Work out the finished part from the listing and answer in its coordinate system (mm). Face numbers are marked on the shaded views. A direction names the side the tool comes from. Give positions to 0.01 mm unless a question says otherwise; leave off trailing zeros. Loops run counter-clockwise (first coordinate to the right, second up) from the corner with the lowest first, then second, coordinate; pieces in that order, holes last. Notation, with made-up numbers: (-5, 12.25) - (1, 12.25) arc R19 ccw to (1, 24.25) - close; hole circle Ø5 at (14, -4.75). An arc over 180 degrees is marked (long way). One line per question, with ' | ' between items. Start each with the question number.
1. For a pull along X with two mould halves and no side action, classify the marked faces 4, 5 and 6 as released by +X, released by -X, zero draft, split by the parting line, or undercut.
2. Section B-B (y = 2.3) is taken. Determine the outline of the cut face in (x, z).
3. Find the intervals of material crossed by line 1 (Z direction, x = -28, y = 1.05); line 2 (Z direction, x = -18, y = 1.95); line 3 (X direction, y = 1.15, z = -0.5), in increasing order.
4. Which of the six approach directions +Z, -Z, +X, -X, +Y, -Y give full straight-line access (tool end or side, diameter ignored) to the marked faces 1, 2 and 3?
5. Each of these flat-tipped pins is pushed along its axis until it touches: pin 1 (0.8 mm diameter, centred on y = 2, z = 3.5, fed in from +X); pin 2 (0.8 mm diameter, centred on y = 1, z = 4.5, fed in from -X); pin 3 (1.8 mm diameter, centred on x = -8, z = 0, fed in from -Y); pin 4 (1.5 mm diameter, centred on x = -2, y = 1, fed in from +Z). Where does it stop, or does it pass through?
6. Section A-A (x = -18) is taken. Determine the outline of the cut face in (y, z), plus the area to 3 significant figures.
7. Section C-C (x = -8) is taken. Determine the outline of the cut face in (y, z).
Autodesk Inventor part; units mm, degrees
ref_plane "YZ Plane" through (0, 0, 0) normal (1, 0, 0) x (0, 1, 0)
ref_plane "XZ Plane" through (0, 0, 0) normal (0, 1, 0) x (-1, 0, 0)
ref_plane "XY Plane" through (0, 0, 0) normal (0, 0, 1) x (1, 0, 0)
sketch "Sketch1" plane through (0, 0, 0) normal (0, 1, 0) x (-1, 0, 0)
  line L0 (0, 0) -> (0, -3)
  line L1 (0, -3) -> (3, -3)
  line L2 (3, -3) -> (3, -5.5)
  line L3 (3, -5.5) -> (33, -5.5)
  line L4 (33, -5.5) -> (33, -3)
  line L5 (33, -3) -> (36, -3)
  line L6 (36, -3) -> (36, 3)
  line L7 (36, 3) -> (33, 3)
  line L8 (33, 3) -> (33, 5.5)
  line L9 (33, 5.5) -> (3, 5.5)
  line L10 (3, 5.5) -> (3, 3)
  line L11 (3, 3) -> (0, 3)
  line L12 (0, 3) -> (0, 0)
  circle A0 centre (28, 0) radius 1.5
  line L13 (0, 0) -> (8, 0)
  circle A1 centre (8, 0) radius 1.5
  arc A2 (17, -1.25) -> (19, -1.25) centre (18, -1.25) ccw
  arc A3 (19, 1.25) -> (17, 1.25) centre (18, 1.25) ccw
  line L14 (19, -1.25) -> (19, 1.25)
  line L15 (17, 1.25) -> (17, -1.25)
  arc A4 (22, -1.25) -> (24, -1.25) centre (23, -1.25) ccw
  arc A5 (24, 1.25) -> (22, 1.25) centre (23, 1.25) ccw
  line L16 (24, -1.25) -> (24, 1.25)
  line L17 (22, 1.25) -> (22, -1.25)
  dimension "d15" = 3
  dimension "d16" = 3
  dimension "d17" = 2.5
  dimension "d18" = 30
  dimension "d19" = 3
  dimension "d20" = 6
  dimension "d21" = 2.5
  dimension "d22" = 30
  dimension "d26" = 8
  dimension "d27" = 3
  dimension "d31" = 8
  dimension "d34" = 1
  dimension "d35" = 11
  dimension "d36" = 20
  dimension "d38" = 1
extrude "Extrusion1" add sketch "Sketch1" along normal blind 3
properties part number "Laser Mount Plate" material "Polycarbonate, Smoke"
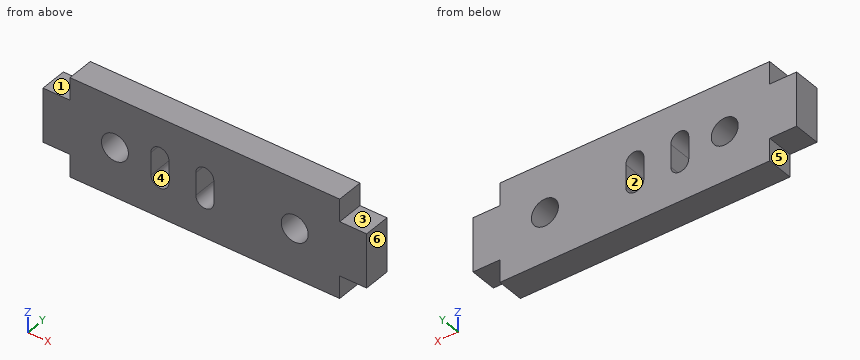
Conclusion:
1) face 4: undercut | face 5: released by -X | face 6: released by +X
2) outline: (-36, -3) - (-33, -3) - (-33, -5.5) - (-3, -5.5) - (-3, -3) - (0, -3) - (0, 3) - (-3, 3) - (-3, 5.5) - (-33, 5.5) - (-33, 3) - (-36, 3) - close; hole circle Ø3 at (-28, 0); hole (-24, -1.25) arc R1 ccw to (-22, -1.25) - (-22, 1.25) arc R1 ccw to (-24, 1.25) - close; hole (-19, -1.25) arc R1 ccw to (-17, -1.25) - (-17, 1.25) arc R1 ccw to (-19, 1.25) - close; hole circle Ø3 at (-8, 0)
3) line 1: -5.5 to -1.5, 1.5 to 5.5 | line 2: -5.5 to -2.25, 2.25 to 5.5 | line 3: -36 to -29.41, -26.59 to -24, -22 to -19, -17 to -9.41, -6.59 to 0
4) face 1: +Z, -X, +Y, -Y | face 2: +Y, -Y | face 3: +Z, +X, +Y, -Y
5) pin 1: x = -3 | pin 2: x = -33 | pin 3: through | pin 4: z = 3
6) outline: (0, -5.5) - (3, -5.5) - (3, -2.25) - (0, -2.25) - close; (0, 2.25) - (3, 2.25) - (3, 5.5) - (0, 5.5) - close | area: 19.5 mm²
7) outline: (0, -5.5) - (3, -5.5) - (3, -1.5) - (0, -1.5) - close; (0, 1.5) - (3, 1.5) - (3, 5.5) - (0, 5.5) - close
